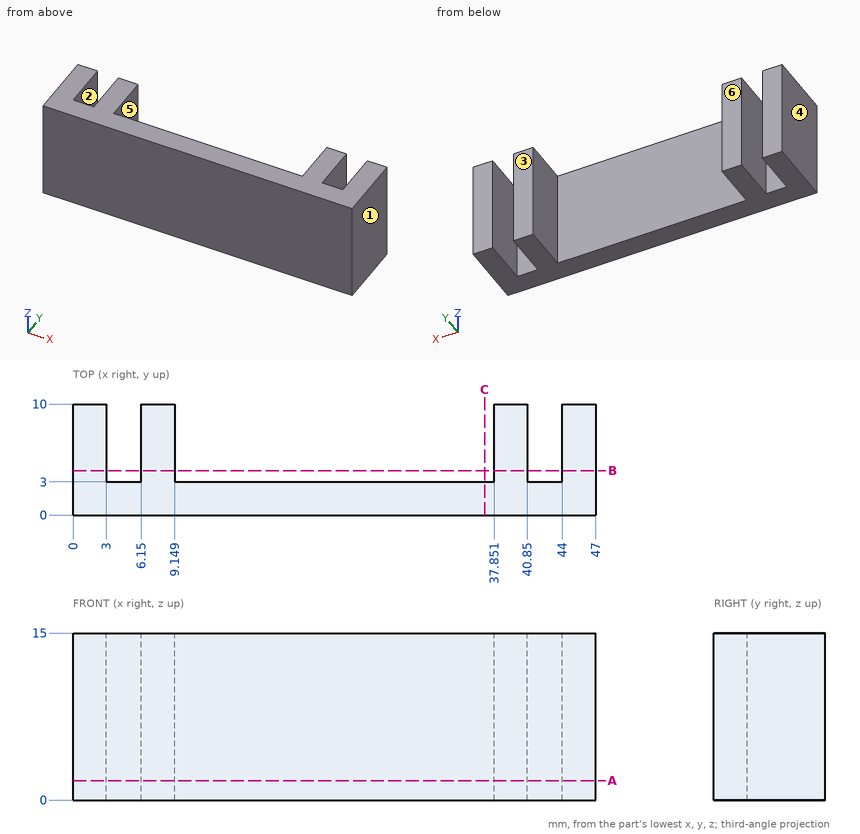
Source: three-view drawing plus pictorial views. Frame: mm from the lowest corner of the part. A direction names the side the tool comes from. Give positions to 0.01 mm unless a question says otherwise; leave off trailing zeros. Loops run counter-clockwise (first coordinate to the right, second up) from the corner with the lowest first, then second, coordinate; pieces in that order, holes last. Notation, with made-up numbers: M 87.25,-19 L 92.25,-19 A28 cw 92.25,20 Z; hole C -38,-9.75 d1. An arc over 180 degrees is marked long. Use CSV: the item, a comma, the result in double quotes.
(1) Pin query (flat end, axial travel): P1, Ø2.5, axis at x = 42.5, z = 10.5, coming from the +Y side. Return the tip coordinate at first contact, or that it passes through.
Outcome:
P1,"stops at y = 3"
(2) Set-up query: the marked faces 5 and 6. Return all of +Z, -Z, +X, -X, +Y, -Y with unobstructed straight access to the full face (end or side cutting, diameter ignored); none if empty.
Outcome:
face 5,"+Z, -Z, +Y"
face 6,"+Z, -Z, +X, -X, +Y"
(3) Section C-C, the plane x = 37. Return loops of the section in (y, z).
Outcome:
outline,"M 0,0 L 3,0 L 3,15 L 0,15 Z"
(4) Section B-B, the plane y = 4. Return loops of the section in (x, z).
Outcome:
outline,"M 0,0 L 3,0 L 3,15 L 0,15 Z; M 6.15,0 L 9.15,0 L 9.15,15 L 6.15,15 Z; M 37.85,0 L 40.85,0 L 40.85,15 L 37.85,15 Z; M 44,0 L 47,0 L 47,15 L 44,15 Z"
(5) Section A-A, the plane z = 1.75. Return loops of the section in (x, y).
Outcome:
outline,"M 0,0 L 47,0 L 47,10 L 44,10 L 44,3 L 40.85,3 L 40.85,10 L 37.85,10 L 37.85,3 L 9.15,3 L 9.15,10 L 6.15,10 L 6.15,3 L 3,3 L 3,10 L 0,10 Z"
(6) Pull-direction query (X, two-part tool) for the marked faces 1, 2, 3 and 4; classes: pulls with the +X half, pulls with the -X half, needs draft (parallel to the pull), parting line crosses it, or undercut.
Outcome:
face 1,"pulls with the +X half"
face 2,"undercut"
face 3,"needs draft"
face 4,"pulls with the -X half"
(7) Material intervals for L1, parallel to X at y = 6.75, z = 4.5; L2, parallel to Y at x = 35.5, z = 12.25, sorted ascending. Write a range as [from, to].
Outcome:
L1,"x = [0, 3], [6.15, 9.15], [37.85, 40.85], [44, 47]"
L2,"y = [0, 3]"
